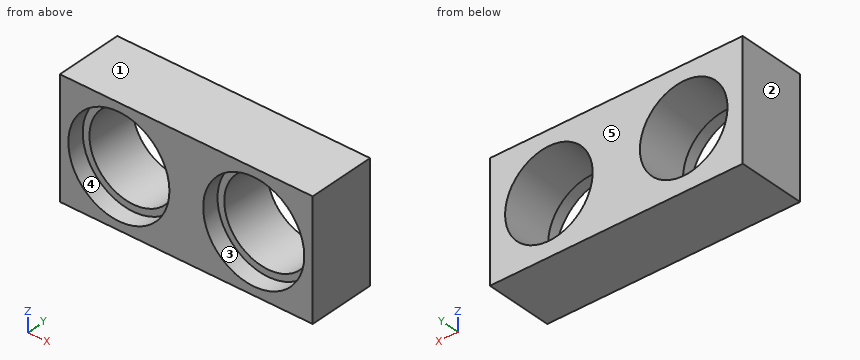
```python
from build123d import *

# Parameters (mm, degrees)
CROQUIS1_W              = 15
CROQUIS1_H              = 7
CROQUIS1_R              = 2.6
SALIENTE_EXTRUIR1_DEPTH = 4
CROQUIS2_R              = 3
CORTAR_EXTRUIR1_DEPTH   = 1


with BuildPart() as part:
    # Croquis1 → Saliente-Extruir1 (new body)
    with BuildSketch(Plane(origin=(0, 0, 0), x_dir=(1, 0, 0), z_dir=(0, 1, 0))):
        with Locations((-4, 0)):
            Rectangle(CROQUIS1_W, CROQUIS1_H)
        Circle(CROQUIS1_R, mode=Mode.SUBTRACT)
        with Locations((-8, 0)):
            Circle(CROQUIS1_R, mode=Mode.SUBTRACT)
    extrude(amount=SALIENTE_EXTRUIR1_DEPTH)

    # Croquis2 → Cortar-Extruir1 (cut)
    with BuildSketch(Plane.XZ):
        Circle(CROQUIS2_R)
        with Locations((-8, 0)):
            Circle(CROQUIS2_R)
    extrude(amount=-CORTAR_EXTRUIR1_DEPTH, mode=Mode.SUBTRACT)


solid = part.part
```
Design review of the part built by this model. Coordinates are the model's own, in mm. Face numbers are marked on the shaded views. A direction names the side the tool comes from. Coordinates: 2 decimals unless noted, no trailing zeros. Write each loop counter-clockwise with the first axis right and the second up, starting at its lowest first coordinate (ties: lowest second). Pieces come first, ordered by that corner, then holes.
1) Mouldability with a two-part tool opening along X and no side actions: class the marked faces 1, 2 and 3 as +X half, -X half, draft (parallel to the pull), parting line (faces both ways), or undercut.
2) Add section A-A (z = 0). Write out the cut boundary in (x, y).
3) Add section B-B (x = 0). Write out the cut boundary in (y, z), plus the area to 3 significant figures.
4) Add section D-D (x = -9.5). Write out the cut boundary in (y, z).
5) To check wall thickness, follow L1, parallel to X at y = 3, z = 0; L2, parallel to Z at x = -8, y = 1.9; L3, parallel to Z at x = -8, y = 0.65. State the ranges of each line that lie inside material, in increasing order.
6) Machinability: for the marked faces 4 and 5, which of the approach directions +Z, -Z, +X, -X, +Y, -Y give a long, thin tool a straight path to every point of the face, cutting with its end or side? Answer none if there is none.
7) Add section C-C (y = 3.4). Write out the cut boundary in (x, z), plus the area to 3 significant figures.
Check result:
1. face 1: draft
1. face 2: -X half
1. face 3: undercut
2. outline: (-11.5, 0) - (-11, 0) - (-11, 1) - (-10.6, 1) - (-10.6, 4) - (-11.5, 4) - close; (-5.4, 1) - (-5, 1) - (-5, 0) - (-3, 0) - (-3, 1) - (-2.6, 1) - (-2.6, 4) - (-5.4, 4) - close; (2.6, 1) - (3, 1) - (3, 0) - (3.5, 0) - (3.5, 4) - (2.6, 4) - close
3. outline: (0, -3.5) - (4, -3.5) - (4, -2.6) - (1, -2.6) - (1, -3) - (0, -3) - close; (0, 3) - (1, 3) - (1, 2.6) - (4, 2.6) - (4, 3.5) - (0, 3.5) - close
3. area: 6.40 mm2
4. outline: (0, -3.5) - (4, -3.5) - (4, -2.12) - (1, -2.12) - (1, -2.6) - (0, -2.6) - close; (0, 2.6) - (1, 2.6) - (1, 2.12) - (4, 2.12) - (4, 3.5) - (0, 3.5) - close
5. L1: x = -11.5 to -10.6, -5.4 to -2.6, 2.6 to 3.5
5. L2: z = -3.5 to -2.6, 2.6 to 3.5
5. L3: z = -3.5 to -3, 3 to 3.5
6. face 4: -Y
6. face 5: +Z, -Z, +X, -X, +Y
7. outline: (-11.5, -3.5) - (3.5, -3.5) - (3.5, 3.5) - (-11.5, 3.5) - close; hole circle Ø5.2 at (-8, 0); hole circle Ø5.2 at (0, 0)
7. area: 62.5 mm2
